Read the model definition and answer for the solid it produces. Units are mm, in the model's axes. Face numbers are marked on the shaded views. Coordinates: 2 decimals unless noted, no trailing zeros. Loops run counter-clockwise (first coordinate to the right, second up) from the corner with the lowest first, then second, coordinate; pieces in that order, holes last. Notation, with made-up numbers: (-25.75, 64.5) -> (-9.75, 64.5) arc R32 cw to (-9.75, 90.5) -> close; hole circle Ø6 at (35.25, 62.5). An arc over 180 degrees is marked (long way). Answer in a Markdown table with one row per item.
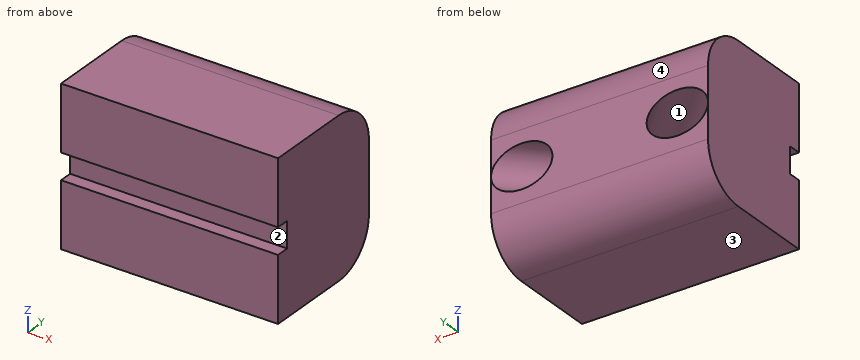
```python
from build123d import *

# Parameters (mm, degrees)
F0_W     = 50
F0_H     = 36
F1_DEPTH = 30
F4_D     = 10
F4_DEPTH = 20
F4_START = 10
F4_TIP   = 3.0043030951
F7_D     = 10
F7_DEPTH = 20
F7_START = 10
F7_TIP   = 3.0043030951
F8_W     = 50
F8_H     = 6
F9_DEPTH = 3
F10_R    = 10


with BuildPart() as f1:
    # F0 (on Front) → F1 (new body)
    with BuildSketch(Plane.XZ):
        Rectangle(F0_W, F0_H)
    extrude(amount=F1_DEPTH)

    # F4
    # its depths count from where the whole tool has entered the part; down to there all is cleared
    with Locations(Plane(origin=(-12.5, 12.5, 0), x_dir=(-0.7071067812, -0.7071067812, 0), z_dir=(-0.7071067812, 0.7071067812, 0)).offset(-F4_START)):
        with Locations((12.6776695297, 0)):
            Hole(F4_D / 2, depth=F4_DEPTH)
            with Locations((0, 0, -(F4_DEPTH + F4_TIP / 2))):  # 118° drill point
                Cone(0, F4_D / 2, F4_TIP, mode=Mode.SUBTRACT)

    # F7
    # its depths count from where the whole tool has entered the part; down to there all is cleared
    with Locations(Plane(origin=(12.5, 12.5, 0), x_dir=(-0.7071067812, 0.7071067812, 0), z_dir=(0.7071067812, 0.7071067812, 0)).offset(-F7_START)):
        with Locations((-12.6776695297, 0)):
            Hole(F7_D / 2, depth=F7_DEPTH)
            with Locations((0, 0, -(F7_DEPTH + F7_TIP / 2))):  # 118° drill point
                Cone(0, F7_D / 2, F7_TIP, mode=Mode.SUBTRACT)

    # F8 (on face) → F9 (cut)
    with BuildSketch(Plane.XZ.offset(30)):
        Rectangle(F8_W, F8_H)
    extrude(amount=-F9_DEPTH, mode=Mode.SUBTRACT)

    # F10
    f10_edges = [f1.edges().sort_by_distance(p)[0] for p in [
        (0, 0, -18),
        (0, 0, 18),
    ]]
    fillet(f10_edges, radius=F10_R)


solid = f1.part
```
1. Given pin 1 Ø1 at (x, y) = (11.5, -8) entering from +Z, flat-ended and moving along its own axis, determine where the tip first touches the part or whether it passes through.
A:
| item | result |
|---|---|
| pin 1 | stops at z = 17.89 |
2. The mould has two halves that part along Z. Classify the marked faces 1, 2, 3 and 4: pulls with the +Z half, pulls with the -Z half, needs draft (parallel to the pull), parting line crosses it, or undercut.
A:
| item | result |
|---|---|
| face 1 | undercut |
| face 2 | undercut |
| face 3 | pulls with the -Z half |
| face 4 | pulls with the +Z half |
3. A cutting plane is placed at A-A on z = -11.5. Give the vertices of the cut face in (x, y).
A:
| item | result |
|---|---|
| outline | (-25, -30) -> (25, -30) -> (25, -0.63) -> (-25, -0.63) -> close |
4. Find the intervals of material crossed by probe 1 along Y at (x, z) = (-1, -1); probe 2 along Z at (x, y) = (-15, -4.75); probe 3 along X at (y, z) = (-18.5, 3.5), in increasing order.
A:
| item | result |
|---|---|
| probe 1 | y = -27 to -20.41, -10 to 0 |
| probe 2 | z = -16.51 to -4.83, 4.83 to 16.51 |
| probe 3 | x = -25 to -4.48, 4.48 to 25 |
5. A cutting plane is placed at B-B on y = -2. Count the separate pieces of the cut face and the enclosed holes in it, and give its area (3 significant figures).
A:
| item | result |
|---|---|
| separate pieces | 1 |
| enclosed holes | 2 |
| area | 1,180 mm2 |
